Geometry check sheet. Reference: the model listing, model coordinates, mm. Face numbers are marked on the shaded views. Round coordinates to 2 decimals unless told otherwise and drop trailing zeros. Order: outer loops, then holes, each group sorted by start corner. A loop starts at its lowest first (then second) coordinate and runs counter-clockwise, first axis right, second up.
(1) Gauge pin test, flat ends, axial feed: P1, Ø3, axis at x = 9.4, y = 0, coming from the -Z side; P2, Ø5.5, axis at y = 0, z = 0, coming from the -X side; P3, Ø2, axis at x = 14.5, z = 1.5, coming from the -Y side; P4, Ø1.5, axis at x = 11, y = -3.5, coming from the -Z side. Record the tip position at first contact, or that the pin passes through.
(2) Cross-section at B-B on y = 0. Enter the section's corners in (x, z).
(3) Cross-section at C-C on x = 7.5. Enter the section's corners in (y, z).
(4) Draft check along Z on the marked faces 1 and 2. Enter one of: pulls with the +Z half, pulls with the -Z half, needs draft (parallel to the pull), parting line crosses it, or undercut.
(5) Thickness scan on L1, parallel to Y at x = 11.5, z = 0; L2, parallel to Y at x = 0.5, z = 0; L3, parallel to X at y = -3.5, z = 0. Record the ranges inside material, lowest first.
(6) Cross-section at A-A on z = 0. Enter the section's corners in (x, y), and give its area (3 significant figures).
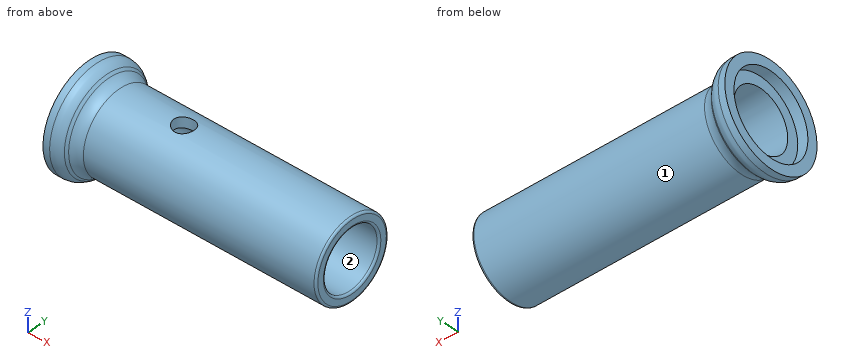
from build123d import *

# Parameters (mm, degrees)
ESQUISSE4_W = 1
ESQUISSE4_H = 5.05


with BuildPart() as part:
    # Esquisse1 → Révolution1 (revolve)
    with BuildSketch(Plane.XY, mode=Mode.PRIVATE) as r_volution1_sk:
        with BuildLine():
            Line((0, 4.05), (0, 5.05))
            Line((0, 5.05), (0.657359313, 5.05))
            ThreePointArc((0.657359313, 5.05), (1.231384461, 4.935819299), (1.718019485, 4.610660172))
            Line((1.718019485, 4.610660172), (1.939339828, 4.389339828))
            ThreePointArc((1.939339828, 4.389339828), (2.425974851, 4.064180701), (3, 3.95))
            Line((3, 3.95), (25.8, 3.95))
            ThreePointArc((25.8, 3.95), (25.941421356, 3.891421356), (26, 3.75))
            Line((26, 3.75), (26, 3.15))
            ThreePointArc((26, 3.15), (25.941421356, 3.008578644), (25.8, 2.95))
            Line((25.8, 2.95), (1, 2.95))
            Line((1, 2.95), (1, 4.05))
            Line((1, 4.05), (0, 4.05))
        make_face()
    revolve(r_volution1_sk.sketch.rotate(Axis((-11.300588411, 0, 0), (1, 0, 0)), 90), axis=Axis((-11.300588411, 0, 0), (1, 0, 0)))

    # Esquisse4 → Dégagement M21 (revolve, cut)
    with BuildSketch(Plane.YZ.offset(9.4)):
        with Locations((0.5, 2.525)):
            Rectangle(ESQUISSE4_W, ESQUISSE4_H)
    revolve(axis=Axis((9.4, 0, -6.35), (0, 0, 1)), mode=Mode.SUBTRACT)


solid = part.part
Found:
1. P1: stops at z = -3.95
1. P2: passes through
1. P3: stops at y = -3.92
1. P4: stops at z = -2.84
2. outline: (0, -5.05) - (0.66, -5.05) arc R1.5 ccw to (1.72, -4.61) - (1.94, -4.39) arc R1.5 cw to (3, -3.95) - (25.8, -3.95) arc R0.2 ccw to (26, -3.75) - (26, -3.15) arc R0.2 ccw to (25.8, -2.95) - (1, -2.95) - (1, -4.05) - (0, -4.05) - close; (0, 4.05) - (1, 4.05) - (1, 2.95) - (8.4, 2.95) - (8.4, 3.95) - (3, 3.95) arc R1.5 cw to (1.94, 4.39) - (1.72, 4.61) arc R1.5 ccw to (0.66, 5.05) - (0, 5.05) - close; (10.4, 2.95) - (25.8, 2.95) arc R0.2 ccw to (26, 3.15) - (26, 3.75) arc R0.2 ccw to (25.8, 3.95) - (10.4, 3.95) - close
3. outline: circle Ø7.9 at (0, 0); hole circle Ø5.9 at (0, 0)
4. face 1: parting line crosses it
4. face 2: undercut
5. L1: y = -3.95 to -2.95, 2.95 to 3.95
5. L2: y = -5.05 to -4.05, 4.05 to 5.05
5. L3: x = 1 to 26
6. outline: (0, -5.05) - (0.66, -5.05) arc R1.5 ccw to (1.72, -4.61) - (1.94, -4.39) arc R1.5 cw to (3, -3.95) - (25.8, -3.95) arc R0.2 ccw to (26, -3.75) - (26, -3.15) arc R0.2 ccw to (25.8, -2.95) - (1, -2.95) - (1, -4.05) - (0, -4.05) - close; (0, 4.05) - (1, 4.05) - (1, 2.95) - (25.8, 2.95) arc R0.2 ccw to (26, 3.15) - (26, 3.75) arc R0.2 ccw to (25.8, 3.95) - (3, 3.95) arc R1.5 cw to (1.94, 4.39) - (1.72, 4.61) arc R1.5 ccw to (0.66, 5.05) - (0, 5.05) - close
6. area: 53.8 mm2
